```python
from build123d import *

# Parameters (mm, degrees)
F0_W     = 50
F0_H     = 50
F1_DEPTH = 25
F0_W_2   = 20.7156650722
F0_H_2   = 28.3317221329
F2_DEPTH = 32.8626733273


with BuildPart() as f1:
    # F0 (on Front) → F1 (new body)
    with BuildSketch(Plane.XZ):
        with Locations((3.7886876613, 2.456478402)):
            Rectangle(F0_W, F0_H)
    extrude(amount=F1_DEPTH)



with BuildPart() as f1b:
    # F0 (on Front) → F1, piece 2 (new body)
    with BuildSketch(Plane.XZ):
        with Locations((-64.4318182021, 2.8941002674)):
            Rectangle(F0_W_2, F0_H_2)
    extrude(amount=F1_DEPTH)


with BuildPart() as f1_1:
    add(f1.part)
    # F2 (add, through all): a face of the model
    f2_faces = [f1b.part.faces().sort_by_distance(p)[0] for p in [
        (-54.073985666, -12.5, 2.8941002674),
    ]]

    add(f1b.part)  # F2 merges F1b
    extrude(f2_faces, amount=F2_DEPTH)


solid = f1_1.part
```
Model file for the job. Use its own axes, mm. A direction names the side the tool comes from. Round coordinates to 2 decimals unless told otherwise and drop trailing zeros. Write each loop counter-clockwise with the first axis right and the second up, starting at its lowest first coordinate (ties: lowest second). Pieces come first, ordered by that corner, then holes. Notation, with made-up numbers: (-3, 39) -> (29, 39) arc R13 ccw to (29, 51) -> close; hole circle Ø10 at (-0.5, -18). An arc over 180 degrees is marked (long way). Answer as CSV lines item,"result".
1. Slice it at C-C, the plane x = -54. List the corners of the cut face in (y, z).
Resolved:
outline,"(-25, -11.27) -> (0, -11.27) -> (0, 17.06) -> (-25, 17.06) -> close"
2. Tool access for faces 1 (the face through (28.789, -12, 2)), 2 (the face through (-48, -12, 17.06)), 3 (the face through (-21.211, -12, -17)): list every direction of +Z, -Z, +X, -X, +Y, -Y with a clear straight run to the whole face (end or side of a thin tool).
Resolved:
face 1,"+Z, -Z, +X, +Y, -Y"
face 2,"+Z, -X, +Y, -Y"
face 3,"-Z, -X, +Y, -Y"
3. Pin check, flat tips, straight feed: pin 1 Ø2 at (y, z) = (-20, 20) entering from -X; pin 2 Ø1 at (x, y) = (-53, -10) entering from -Z; pin 3 Ø3 at (x, z) = (-40, -7) entering from +Y. Stop position of each tip, or through.
Resolved:
pin 1,"x = -21.21"
pin 2,"z = -11.27"
pin 3,"y = 0"
4. Drill centre lines: line 1 (Z direction, x = -62.5, y = -16); line 2 (X direction, y = -18, z = -13). Where is each one in solid material? Low to high.
Resolved:
line 1,"-11.27 to 17.06"
line 2,"-21.21 to 28.79"
5. Slice it at A-A, the plane y = -3.5. List the corners of the cut face in (x, z).
Resolved:
outline,"(-74.79, -11.27) -> (-21.21, -11.27) -> (-21.21, -22.54) -> (28.79, -22.54) -> (28.79, 27.46) -> (-21.21, 27.46) -> (-21.21, 17.06) -> (-74.79, 17.06) -> close"
6. Slice it at B-B, the plane z = 22. List the corners of the cut face in (x, y), plus the area to 3 significant figures.
Resolved:
outline,"(-21.21, -25) -> (28.79, -25) -> (28.79, 0) -> (-21.21, 0) -> close"
area,"1,250 mm²"
